Part model, mm, in its own coordinate system. A direction names the side the tool comes from. Round coordinates to 2 decimals unless told otherwise and drop trailing zeros. Write each loop counter-clockwise with the first axis right and the second up, starting at its lowest first coordinate (ties: lowest second). Pieces come first, ordered by that corner, then holes. Notation, with made-up numbers: (-2.75, -4) -> (18.25, -4) arc R12 cw to (18.25, 15) -> close; hole circle Ø6 at (-38.5, 5.25). An arc over 180 degrees is marked (long way). Return JSON: item names as keys, results as strings. Group by question number.
(1) Drill centre lines: L1, parallel to Z at x = 0, y = -0.25; L2, parallel to Z at x = 0, y = 11; L3, parallel to X at y = 4, z = 0. Where is each one in solid material? Low to high. Write a range as from..to.
(2) Tool access for faces 1 (the flat face through (-7, 22, -4)), 2 (the cylindrical face through (-4.88, 5.87, -1.08)): list every direction of +Z, -Z, +X, -X, +Y, -Y with a clear straight run to the whole face (end or side of a thin tool).
(3) Mould opens along X. For faces 3 (the flat face through (-7, 24, -4)), 4 (the cylindrical face through (6.93, 10.75, 2.87)), 5 (the flat face through (2, 20, 5)) say: +X half, -X half, draft (parallel to the pull), parting line (faces both ways), or undercut.
(4) Drop flat-ended pins along their axis: pin 1 Ø4 at (x, y) = (-5, 17.5) entering from -Z; pin 2 Ø4 at (y, z) = (8, -7.5) entering from +X; pin 3 Ø4.5 at (x, z) = (-3.5, -3.5) entering from +Y. Give the stop position or say it passes through.
(5) Saw through at B-B (y = 4). List the corners of the cut face in (x, z).
(6) Saw through at A-A (y = 10). List the corners of the cut face in (x, z).
from build123d import *

# Parameters (mm, degrees)
SKETCH_3_R          = 7.5
EXTRUDE_1_DEPTH     = 20
SKETCH_5_R          = 5
CUT_EXTRUDE_1_DEPTH = 34.166247904


with BuildPart() as part:
    # 扫描1: sweep along a path in 草图2
    with BuildLine(Plane(origin=(0, 0, 0), x_dir=(1, 0, 0), z_dir=(0, 1, 0))) as sweep_1_path:
        CenterArc((0, 0), 10, 0, 360)
    # 草图1 → 扫描1 (sweep)
    with BuildSketch(Plane.XY):
        with BuildLine():
            Line((0, 10), (0, -10))
            ThreePointArc((0, -10), (10, 0), (0, 10))
        make_face()
    sweep(path=sweep_1_path.line)

    # 草图3 → 凸台-拉伸1 (add)
    with BuildSketch(Plane(origin=(0, 0, 0), x_dir=(1, 0, 0), z_dir=(0, 1, 0))):
        Circle(SKETCH_3_R)
    extrude(amount=EXTRUDE_1_DEPTH)

    # 扫描2: sweep along a curve in space
    with BuildLine() as sweep_2_path:
        ThreePointArc((0, 20, 7.5), (5.303300859, 20, 5.303300859), (7.5, 20, 0))
        ThreePointArc((7.5, 20, 0), (5.303300859, 20, -5.303300859), (0, 20, -7.5))
        ThreePointArc((0, 20, -7.5), (-5.303300859, 20, -5.303300859), (-7.5, 20, 0))
        ThreePointArc((-7.5, 20, 0), (-5.303300859, 20, 5.303300859), (0, 20, 7.5))
    # 草图4 → 扫描2 (sweep)
    with BuildSketch(Plane.XY):
        Polygon((7.5, 22), (8.3, 22), (7.5, 20), (7.5, 15), (9, 20), (9, 24), (7.5, 24), align=None)
    sweep(path=sweep_2_path.line)

    # 草图5 → 切除-拉伸1 (cut, through all)
    with BuildSketch(Plane(origin=(0, 20, 0), x_dir=(1, 0, 0), z_dir=(0, 1, 0))):
        with Locations(Location((0, 0, 0), (0, 0, 270))):
            Circle(SKETCH_5_R)
    extrude(amount=-CUT_EXTRUDE_1_DEPTH, mode=Mode.SUBTRACT)


solid = part.part
Computed values:
{
 "1": {"L1": "-10..-5, 5..10", "L2": "-7.5..-5, 5..7.5", "L3": "-9.17..-5, 5..9.17"},
 "2": {"face 1": "none", "face 2": "+Y, -Y"},
 "3": {"face 3": "draft", "face 4": "parting line", "face 5": "undercut"},
 "4": {"pin 1": "z = -7.91", "pin 2": "x = 5.1", "pin 3": "y = 20"},
 "5": {"outline": "circle Ø18.33 at (0, 0); hole circle Ø10 at (0, 0)"},
 "6": {"outline": "circle Ø15 at (0, 0); hole circle Ø10 at (0, 0)"}
}
